Verification items for the finished model (mm, model axes). A direction names the side the tool comes from. Coordinates: 2 decimals unless noted, no trailing zeros. Order: outer loops, then holes, each group sorted by start corner. A loop starts at its lowest first (then second) coordinate and runs counter-clockwise, first axis right, second up. Notation, with made-up numbers: (43, -32) - (52, -32) arc R22 ccw to (52, -22) - close; hole circle Ø7 at (39.5, 70.25). An arc over 180 degrees is marked (long way). Answer as CSV lines item,"result". Start each with the question number.
1. Section check D-D (y = 80). Record the cut outline in (x, z), and give its area (3 significant figures).
2. Material ranges on L1, parallel to Y at x = 38, z = -7; L2, parallel to Z at x = 10, y = 112; L3, parallel to X at y = 63, z = -12.75, recorded low to high. Write a range as [from, to].
3. Section check A-A (z = 7.5). Record the cut outline in (x, y), and give its area (3 significant figures).
4. Section check B-B (x = 10). Record the cut outline in (y, z).
5. Set-up check for faces 1 (the flat face through (21, 111.512, 0)), 2 (the cylindrical face through (0.8, 16.6, -8.52)): record each of +Z, -Z, +X, -X, +Y, -Y from which the full face is reachable in a straight line by a thin tool's end or side.
6. Mould release check, pull along Z, two halves, no side actions. Record for faces 3 (the flat face through (20, 113.1, 0)), 4 (the cylindrical face through (0.8, 16.6, 6.48)), 5 (the cylindrical face through (11.897, 112.295, -0.083)), 6 (the flat face through (1, 57, 15)): pulls with the +Z half, pulls with the -Z half, needs draft (parallel to the pull), parting line crosses it, or undercut.
7. Section check C-C (z = 0). Record the cut outline in (x, y), and give its area (3 significant figures).
8. Go/stop test with flat-tipped pins: pin 1 (1 mm diameter, centred on y = 41.5, z = 6, fed in from +X); pin 2 (1 mm diameter, centred on x = 29.5, z = -3, fed in from -Y). Record where each tip stops, or that it passes through.
from build123d import *

# Parameters (mm, degrees)
BOSS_EXTRUDE1_DEPTH   = 15
F_6_CLEARANCE_HOLE1_D = 3.7973
F_6_CLEARANCE_HOLE2_D = 3.7973


with BuildPart() as part:
    # Sketch1 → Boss-Extrude1 (new, symmetric)
    with BuildSketch(Plane.XY):
        Polygon((0, 0), (0, 113.1), (40, 113.1), (40, 111.5125), (1.5875, 111.5125), (1.5875, 0), align=None)
    extrude(amount=BOSS_EXTRUDE1_DEPTH, both=True)

    # #6 Clearance Hole1 (through all)
    with Locations(Plane.ZY):
        with Locations((-7.5, 15), (7.5, 15)):
            Hole(F_6_CLEARANCE_HOLE1_D / 2)

    # #6 Clearance Hole2 (through all)
    with Locations(Plane(origin=(0, 113.1, 0), x_dir=(1, 0, 0), z_dir=(0, 1, 0))):
        with Locations((10, 0), (30, 0)):
            Hole(F_6_CLEARANCE_HOLE2_D / 2)


solid = part.part
Evaluation:
1,outline,"(0, -15) - (1.59, -15) - (1.59, 15) - (0, 15) - close"
1,area,"47.6 mm²"
2,L1,"y = [111.51, 113.1]"
2,L2,"z = [-15, -1.9], [1.9, 15]"
2,L3,"x = [0, 1.59]"
3,outline,"(0, 0) - (1.59, 0) - (1.59, 13.1) - (0, 13.1) - close; (0, 16.9) - (1.59, 16.9) - (1.59, 111.51) - (40, 111.51) - (40, 113.1) - (0, 113.1) - close"
3,area,"234 mm²"
4,outline,"(111.51, -15) - (113.1, -15) - (113.1, -1.9) - (111.51, -1.9) - close; (111.51, 1.9) - (113.1, 1.9) - (113.1, 15) - (111.51, 15) - close"
5,face 1,"+Z, -Z, +X, -Y"
5,face 2,"+X, -X"
6,face 3,"needs draft"
6,face 4,"undercut"
6,face 5,"undercut"
6,face 6,"pulls with the +Z half"
7,outline,"(0, 0) - (1.59, 0) - (1.59, 111.51) - (8.1, 111.51) - (8.1, 113.1) - (0, 113.1) - close; (11.9, 111.51) - (28.1, 111.51) - (28.1, 113.1) - (11.9, 113.1) - close; (31.9, 111.51) - (40, 111.51) - (40, 113.1) - (31.9, 113.1) - close"
7,area,"228 mm²"
8,pin 1,"stops at x = 1.59"
8,pin 2,"stops at y = 111.51"
